from build123d import *

# Parameters (mm, degrees)
CROQUIS1_R                 = 21
SALIENTE_EXTRUIR1_DEPTH    = 7.5
CROQUIS2_R                 = 14.95
SALIENTE_EXTRUIR2_DEPTH    = 20
CORTAR_EXTRUIR1_DEPTH      = 41.475301111
CORTAR_EXTRUIR1_DEPTH_BACK = 2.5
CORTAR_EXTRUIR2_DEPTH      = 39.820097888
CORTAR_EXTRUIR2_DEPTH_BACK = 1.5
CROQUIS4_R                 = 5.5


with BuildPart() as part:
    # Croquis1 → Saliente-Extruir1 (new body)
    with BuildSketch(Plane(origin=(0, 0, 0), x_dir=(1, 0, 0), z_dir=(0, 1, 0))):
        with Locations(Location((0, 0, 0), (0, 0, 270))):
            Circle(CROQUIS1_R)
    extrude(amount=SALIENTE_EXTRUIR1_DEPTH)

    # Croquis2 → Saliente-Extruir2 (add)
    with BuildSketch(Plane(origin=(0, 7.5, 0), x_dir=(1, 0, 0), z_dir=(0, 1, 0))):
        with Locations(Location((0, 0, 0), (0, 0, 270))):
            Circle(CROQUIS2_R)
    extrude(amount=SALIENTE_EXTRUIR2_DEPTH)

    # Croquis3 → Cortar-Extruir1 (cut, two sides: drawn at the far end of the back side and taken through both)
    with BuildSketch(Plane.XZ.offset(-CORTAR_EXTRUIR1_DEPTH_BACK)):
        with BuildLine():
            Line((-4.971667622, -4.813784484), (-7.886808716, -5.156697725))
            Line((-7.886808716, -5.156697725), (-17.496587444, -4.741948795))
            ThreePointArc((-17.496587444, -4.741948795), (-20.06167777, -2.359890899), (-18.11936882, 0.552380405))
            Line((-18.11936882, 0.552380405), (-8.868149486, 3.18578214))
            Line((-8.868149486, 3.18578214), (-5.953008392, 3.528695381))
            ThreePointArc((-5.953008392, 3.528695381), (-5.084547102, 4.014240505), (-4.813784484, 4.971667622))
            Line((-4.813784484, 4.971667622), (-5.156697725, 7.886808716))
            Line((-5.156697725, 7.886808716), (-4.741948795, 17.496587444))
            ThreePointArc((-4.741948795, 17.496587444), (-2.359890899, 20.06167777), (0.552380405, 18.11936882))
            Line((0.552380405, 18.11936882), (3.18578214, 8.868149486))
            Line((3.18578214, 8.868149486), (3.528695381, 5.953008392))
            ThreePointArc((3.528695381, 5.953008392), (4.014240505, 5.084547102), (4.971667622, 4.813784484))
            Line((4.971667622, 4.813784484), (7.886808716, 5.156697725))
            Line((7.886808716, 5.156697725), (17.496587444, 4.741948795))
            ThreePointArc((17.496587444, 4.741948795), (20.06167777, 2.359890899), (18.11936882, -0.552380405))
            Line((18.11936882, -0.552380405), (8.868149486, -3.18578214))
            Line((8.868149486, -3.18578214), (5.953008392, -3.528695381))
            ThreePointArc((5.953008392, -3.528695381), (5.084547102, -4.014240505), (4.813784484, -4.971667622))
            Line((4.813784484, -4.971667622), (5.156697725, -7.886808716))
            Line((5.156697725, -7.886808716), (4.741948795, -17.496587444))
            ThreePointArc((4.741948795, -17.496587444), (2.359890899, -20.06167777), (-0.552380405, -18.11936882))
            Line((-0.552380405, -18.11936882), (-3.18578214, -8.868149486))
            Line((-3.18578214, -8.868149486), (-3.528695381, -5.953008392))
            ThreePointArc((-3.528695381, -5.953008392), (-4.014240505, -5.084547102), (-4.971667622, -4.813784484))
        make_face()
    extrude(amount=CORTAR_EXTRUIR1_DEPTH + CORTAR_EXTRUIR1_DEPTH_BACK, mode=Mode.SUBTRACT)

    # Croquis4 → Cortar-Extruir2 (cut, two sides: drawn at the far end of the back side and taken through both)
    with BuildSketch(Plane.XZ.offset(-2.5).offset(-CORTAR_EXTRUIR2_DEPTH_BACK)):
        with Locations(Location((0, 0, 0), (0, 0, 270))):
            Circle(CROQUIS4_R)
    extrude(amount=CORTAR_EXTRUIR2_DEPTH + CORTAR_EXTRUIR2_DEPTH_BACK, mode=Mode.SUBTRACT)


solid = part.part
Model file for the job. Use its own axes, mm. A direction names the side the tool comes from. Give positions to 0.01 mm unless a question says otherwise; leave off trailing zeros. Order: outer loops, then holes, each group sorted by start corner. A loop starts at its lowest first (then second) coordinate and runs counter-clockwise, first axis right, second up. Notation, with made-up numbers: M 1,-6.75 L 60,-6.75 A22 cw 60,1.25 Z; hole C 24.25,42 d6. An arc over 180 degrees is marked long. Write item = value, one per line.
Q1. Tool access for faces 4 (the cylindrical face through (6.31, 3.7, 20.03)), 5 (the flat face through (-3.355, 1.268, -7.431)): list every direction of +Z, -Z, +X, -X, +Y, -Y with a clear straight run to the whole face (end or side of a thin tool).
Derived:
face_4 = +Y, -Y
face_5 = -Y
Q2. Flat gauge pins, fed straight in: pin 1 (10 mm diameter, centred on x = -7.5, y = 24.5, fed in from -Z); pin 2 (6 mm diameter, centred on x = 12, z = 15, fed in from +Y); pin 3 (1.5 mm diameter, centred on x = -14, y = 18.5, fed in from +Z). Where does each tip first touch, or does it go through?
Derived:
pin_1 = -14.74
pin_2 = 7.5
pin_3 = 6.92
Q3. Cut at B-B, the plane y = 6.25. List the corners of the cut face in (x, z).
Derived:
outline = C 0,0 d42
Q4. Two-plate mould, pull along Z, no slides. Class faces 1 (the flat face through (-12.624, 1.268, -4.952)), 2 (the flat face through (5, 0, -5)), 3 (the cylindrical face through (-5.73, 17.36, 13.81)): pulls with the +Z half, pulls with the -Z half, needs draft (parallel to the pull), parting line crosses it, or undercut.
Derived:
face_1 = undercut
face_2 = needs draft
face_3 = parting line crosses it
Q5. Cut at D-D, the plane y = 18.25. List the corners of the cut face in (x, z).
Derived:
outline = C 0,0 d29.9
Q6. Cut at A-A, the plane z = 0. List the corners of the cut face in (x, y).
Derived:
outline = M -21,0 L -19.14,0 L -19.14,2.5 L -5.5,2.5 L -5.5,4 L 5.5,4 L 5.5,2.5 L 19.14,2.5 L 19.14,0 L 21,0 L 21,7.5 L 14.95,7.5 L 14.95,27.5 L -14.95,27.5 L -14.95,7.5 L -21,7.5 Z
Q7. Cut at C-C, the plane x = 0. List the corners of the cut face in (y, z), then the cut area to 3 significant figures.
Derived:
outline = M 0,-21 L 7.5,-21 L 7.5,-14.95 L 27.5,-14.95 L 27.5,14.95 L 7.5,14.95 L 7.5,21 L 0,21 L 0,19.14 L 2.5,19.14 L 2.5,5.5 L 4,5.5 L 4,-5.5 L 2.5,-5.5 L 2.5,-19.14 L 0,-19.14 Z
area = 801 mm2
Q8. Drill centre lines: line 1 (X direction, y = 3.5, z = 0); line 2 (Y direction, x = 2.5, z = -12); line 3 (Y direction, x = 4.5, z = 15). Where is each one in solid material? Low to high. Write a range as [from, to].
Derived:
line_1 = [-21, -5.5], [5.5, 21]
line_2 = [2.5, 27.5]
line_3 = [0, 7.5]
